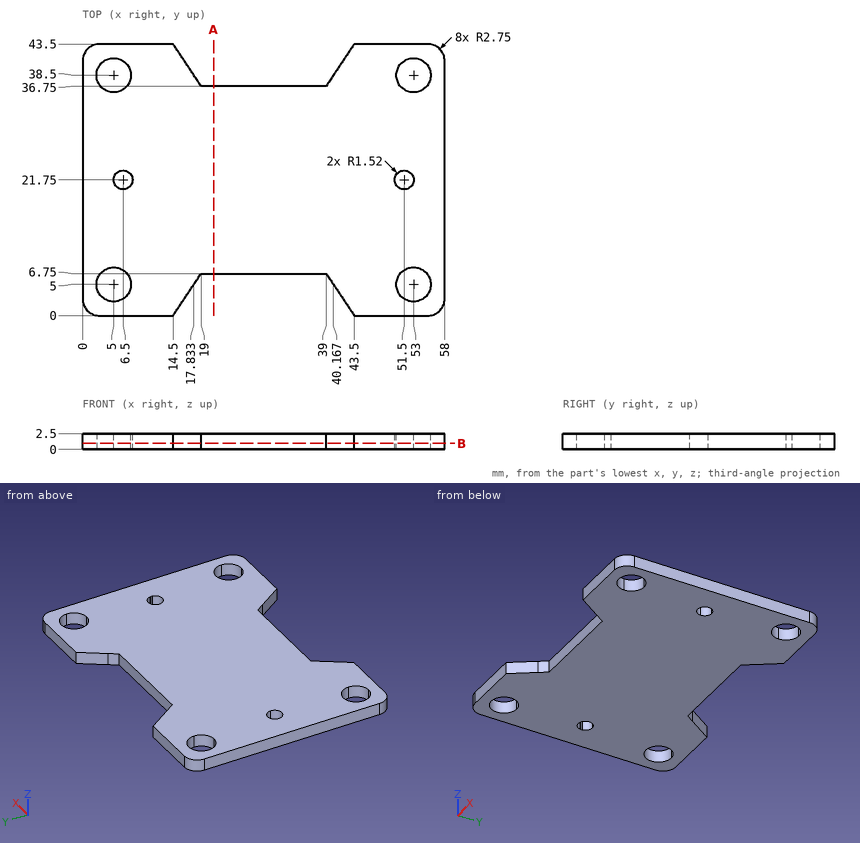
Job drawing, mm, ordinate dimensions from the low corner. One solid piece. Coordinates: 2 decimals unless noted, no trailing zeros. Loops run counter-clockwise (first coordinate to the right, second up) from the corner with the lowest first, then second, coordinate; pieces in that order, holes last. Notation, with made-up numbers: (33.25, 68.5) - (63.25, 68.5) arc R14 ccw to (63.25, 74.5) - close; hole circle Ø2 at (17.5, 2.25). An arc over 180 degrees is marked (long way). Write item = value, one per line. Start each with the question number.
Q1. Drill centre lines: L1, parallel to Y at x = 52, z = 0.2 (1 decimal); L2, parallel to X at y = 7.5, z = 2.2 (1 decimal); L3, parallel to X at y = 4.5, z = 0.45 (1 decimal). Where is each one in solid material? Low to high.
Q2. Flat gauge pins, fed straight in: pin 1 Ø1.5 at (x, y) = (32.5, 38.5) entering from -Z; pin 2 Ø0.8 at (x, z) = (28, 1.5) entering from -Y. Where does each tip first touch, or does it go through?
Q3. Cut at A-A, the plane x = 21. List the corners of the cut face in (y, z).
Q4. Cut at B-B, the plane z = 0.95. List the corners of the cut face in (x, y).
Computed:
q1.L1 = 0 to 2.4, 7.6 to 20.3, 23.2 to 35.9, 41.1 to 43.5
q1.L2 = 0 to 3.9, 6.1 to 51.9, 54.1 to 58
q1.L3 = 0 to 2.3, 7.7 to 17.5, 40.5 to 50.3, 55.7 to 58
q2.pin_1 = through
q2.pin_2 = 6.75
q3.outline = (6.75, 0) - (36.75, 0) - (36.75, 2.5) - (6.75, 2.5) - close
q4.outline = (0, 2.75) arc R2.75 ccw to (2.75, 0) - (14.5, 0) - (19, 6.75) - (39, 6.75) - (43.5, 0) - (55.25, 0) arc R2.75 ccw to (58, 2.75) - (58, 40.75) arc R2.75 ccw to (55.25, 43.5) - (43.5, 43.5) - (39, 36.75) - (19, 36.75) - (14.5, 43.5) - (2.75, 43.5) arc R2.75 ccw to (0, 40.75) - close; hole circle Ø5.5 at (5, 5); hole circle Ø5.5 at (5, 38.5); hole circle Ø3.04 at (6.5, 21.75); hole circle Ø3.04 at (51.5, 21.75); hole circle Ø5.5 at (53, 5); hole circle Ø5.5 at (53, 38.5)
